Autodesk Inventor part; units mm, degrees
ref_plane "YZ Plane" through (0, 0, 0) normal (1, 0, 0) x (0, 1, 0)
ref_plane "XZ Plane" through (0, 0, 0) normal (0, 1, 0) x (-1, 0, 0)
ref_plane "XY Plane" through (0, 0, 0) normal (0, 0, 1) x (1, 0, 0)
sketch "Sketch1" plane through (0, 0, 0) normal (0, 0, 1) x (1, 0, 0)
  line L0 (-18.671, 23.6638) -> (26.829, 23.6638)
  line L1 (26.829, 23.6638) -> (26.829, -28.3362)
  line L2 (26.829, -28.3362) -> (-18.671, -28.3362)
  line L3 (-18.671, -28.3362) -> (-18.671, 23.6638)
  point P0 (0, 0)
  dimension "d0" = 52
  dimension "d1" = 45.5
extrude "Extrusion1" add sketch "Sketch1" along normal blind 2
sketch "Sketch2" plane through (0, 0, 2) normal (0, 0, 1) x (1, 0, 0)
  line L0 (-18.671, -28.3362) -> (26.829, -28.3362)
  line L1 (26.829, -28.3362) -> (26.829, 23.6638)
  line L2 (26.829, 23.6638) -> (-18.671, 23.6638)
  point P0 (0, 0)
  point P1 (-13.171, 20.6638)
  point P2 (21.829, 20.6638)
  point P3 (21.829, -25.3362)
  point P4 (-13.171, -25.3362)
  point P5 (23.829, -28.3362)
  point P6 (26.829, -25.3362)
  point P7 (26.829, 20.6638)
  point P8 (23.829, 23.6638)
  dimension "d5" = 35
  dimension "d6" = 35
  dimension "d7" = 46
  dimension "d8" = 3
  dimension "d9" = 3
  dimension "d10" = 5
  dimension "d11" = 5
  dimension "d12" = 3
hole "Hole1" at (-13.171, 20.6638, 2) at (21.829, 20.6638, 2) at (21.829, -25.3362, 2) at (-13.171, -25.3362, 2) direction (0, 0, -1) diameter 3.2 depth 10 tip angle 118
sketch "Sketch3" plane through (0, 0, 2) normal (0, 0, 1) x (1, 0, 0)
  line L0 (-18.671, 23.6638) -> (-18.671, -28.3362)
  line L1 (-18.671, 15.6638) -> (20.829, 15.6638)
  line L2 (20.829, 15.6638) -> (20.829, -20.3362)
  line L3 (20.829, -20.3362) -> (-18.671, -20.3362)
  line L4 (-18.671, -20.3362) -> (-18.671, 15.6638)
  circle A0 centre (-13.171, 20.6638) radius 1.6
  line L5 (26.829, -28.3362) -> (26.829, 23.6638)
  circle A1 centre (-13.171, -25.3362) radius 1.6
  point P0 (0, 0)
  point P1 (26.829, -25.3362)
  point P2 (26.829, 20.6638)
  dimension "d20" = 5
  dimension "d21" = 6
  dimension "d22" = 5
extrude "Extrusion2" cut sketch "Sketch3" against normal blind 2 contours L1 L2 L3 L0
sketch "Sketch4" plane through (0, 0, 2) normal (0, 0, 1) x (1, 0, 0)
  line L0 (-18.671, 15.6638) -> (20.829, 15.6638)
  line L1 (-18.671, 15.6638) -> (-13.671, 15.6638)
  line L2 (-13.671, 15.6638) -> (-13.671, 7.6638)
  line L3 (-13.671, 7.6638) -> (-18.671, 7.6638)
  line L4 (-18.671, 7.6638) -> (-18.671, 15.6638)
  line L5 (-18.671, -20.3362) -> (-18.671, -28.3362)
  line L6 (-18.671, -20.3362) -> (-13.671, -20.3362)
  line L7 (-13.671, -20.3362) -> (-13.671, -12.3362)
  line L8 (-13.671, -12.3362) -> (-18.671, -12.3362)
  line L9 (-18.671, -12.3362) -> (-18.671, -20.3362)
  point P0 (0, 0)
  point P1 (17.829, 15.6638)
  point P2 (-18.671, -25.3362)
  dimension "d27" = 8
  dimension "d28" = 8
  dimension "d29" = 5
extrude "Extrusion3" add sketch "Sketch4" against normal blind 2
fillet "Fillet5" radius 2 4 edges at (-13.671, 7.6638, 1) (-18.671, 7.6638, 1) (-18.671, -12.3362, 1) (-13.671, -12.3362, 1)
sketch "Sketch5" plane through (0, 0, 2) normal (0, 0, 1) x (1, 0, 0)
  line L0 (26.829, 23.6638) -> (-18.671, 23.6638)
  line L1 (-18.671, 23.6638) -> (26.829, 23.6638)
  line L2 (26.829, 23.6638) -> (26.829, 24.1638)
  line L3 (26.829, 24.1638) -> (-18.671, 24.1638)
  line L4 (-18.671, 24.1638) -> (-18.671, 23.6638)
  line L5 (-18.671, -28.3362) -> (26.829, -28.3362)
  line L6 (-18.671, -28.3362) -> (26.829, -28.3362)
  line L7 (26.829, -28.3362) -> (26.829, -28.8362)
  line L8 (26.829, -28.8362) -> (-18.671, -28.8362)
  line L9 (-18.671, -28.8362) -> (-18.671, -28.3362)
  line L10 (26.829, -28.3362) -> (26.829, 23.6638)
  point P0 (0, 0)
  dimension "d37" = 0.5
  dimension "d38" = 0.5
extrude "Extrusion4" add sketch "Sketch5" against normal blind 2
fillet "Fillet6" radius 3 4 edges at (-18.671, 24.1638, 1) (26.829, 24.1638, 1) (26.829, -28.8362, 1) (-18.671, -28.8362, 1)
chamfer "Chamfer2" distance 3 angle 45 4 edges at (-13.671, 15.6638, 1) (20.829, 15.6638, 1) (-13.671, -20.3362, 1) (20.829, -20.3362, 1)
sketch "Sketch6" plane through (0, 0, 2) normal (0, 0, 1) x (1, 0, 0)
  circle A0 centre (-13.171, -25.3362) radius 1.6
  circle A1 centre (-13.171, 20.6638) radius 1.6
  circle A2 centre (21.829, 20.6638) radius 1.6
  line L0 (23.829, 24.1638) -> (-15.671, 24.1638)
  line L1 (-15.671, -28.8362) -> (23.829, -28.8362)
  circle A3 centre (21.829, -25.3362) radius 1.6
  point P0 (0, 0)
  dimension "d46" = 46
  dimension "d47" = 35
  dimension "d48" = 3.5
  dimension "d49" = 3.5
  dimension "d50" = 3.5
  dimension "d51" = 3.5
properties part number "wood_supp"
Can you work these out from the model? Positions are in its coordinate system, mm. A direction names the side the tool comes from. Round coordinates to 2 decimals unless told otherwise and drop trailing zeros. Order: outer loops, then holes, each group sorted by start corner. A loop starts at its lowest first (then second) coordinate and runs counter-clockwise, first axis right, second up. Notation, with made-up numbers: (86.25, 60) -> (98.25, 60) arc R23 ccw to (98.25, 72) -> close; hole circle Ø1 at (-27.5, -20.75). An arc over 180 degrees is marked (long way). Return JSON: item names as keys, results as strings. Group by question number.
1. We'd pull the mould along X, two halves only. Please class faces 1 (the face through (22.803, 21.934, 0.986)), 2 (the face through (26.829, -2, 1)), 3 (the face through (4, 24.164, 1)): released by +X, released by -X, zero draft, split by the parting line, or undercut.
2. I need wall thicknesses on line 1 (Y direction, x = 8, z = 0.3); line 2 (Y direction, x = -15.5, z = 0.15); line 3 (X direction, y = 12, z = 0.85). Which ranges of each line are inside material? Lowest first, please. Write a range as [from, to].
3. If we section it at D-D, the plane y = 2: Write out the boundary of the cut face in (x, z), then the cut area to 3 significant figures.
4. If we section it at C-C, the plane z = 0.4: Write out the boundary of the cut face in (x, y), then the cut area to 3 significant figures.
5. Which directions (+Z, -Z, +X, -X, +Y, -Y) give clear straight access to the entire face, cutting with the end or side of a thin tool? Please do faces 4 (the face through (4, -20.336, 1)), 5 (the face through (4, 16, 2)).
6. If we section it at A-A, the plane x = 7: Write out the boundary of the cut face in (y, z).
7. If we section it at B-B, the plane y = 20: Write out the boundary of the cut face in (x, z).
8. Will these pins go through, and if not, where does the flat tip stop? pin 1 (1 mm diameter, centred on y = -2.5, z = 0.5, fed in from -X); pin 2 (1.9 mm diameter, centred on x = -13.17, y = 20.66, fed in from +Z).
Output values:
{
 "1": {"face 1": "undercut", "face 2": "released by +X", "face 3": "zero draft"},
 "2": {"line 1": "[-28.84, -20.34], [15.66, 24.16]", "line 2": "[-28.84, -12.34], [7.67, 24.16]", "line 3": "[-18.67, -13.67], [20.83, 26.83]"},
 "3": {"outline": "(20.83, 0) -> (26.83, 0) -> (26.83, 2) -> (20.83, 2) -> close", "area": "12.0 mm²"},
 "4": {"outline": "(-18.67, -25.84) arc R3 ccw to (-15.67, -28.84) -> (23.83, -28.84) arc R3 ccw to (26.83, -25.84) -> (26.83, 21.16) arc R3 ccw to (23.83, 24.16) -> (-15.67, 24.16) arc R3 ccw to (-18.67, 21.16) -> (-18.67, 9.66) arc R2 ccw to (-16.67, 7.66) -> (-15.67, 7.66) arc R2 ccw to (-13.67, 9.66) -> (-13.67, 12.66) -> (-10.67, 15.66) -> (17.83, 15.66) -> (20.83, 12.66) -> (20.83, -17.34) -> (17.83, -20.34) -> (-10.67, -20.34) -> (-13.67, -17.34) -> (-13.67, -14.34) arc R2 ccw to (-15.67, -12.34) -> (-16.67, -12.34) arc R2 ccw to (-18.67, -14.34) -> close; hole circle Ø3.2 at (-13.17, -25.34); hole circle Ø3.2 at (-13.17, 20.66); hole circle Ø3.2 at (21.83, -25.34); hole circle Ø3.2 at (21.83, 20.66)", "area": "1,040 mm²"},
 "5": {"face 4": "+Z, -Z", "face 5": "+Z, +X, -X, +Y, -Y"},
 "6": {"outline": "(-28.84, 0) -> (-20.34, 0) -> (-20.34, 2) -> (-28.84, 2) -> close; (15.66, 0) -> (24.16, 0) -> (24.16, 2) -> (15.66, 2) -> close"},
 "7": {"outline": "(-18.67, 0) -> (-14.63, 0) -> (-14.63, 2) -> (-18.67, 2) -> close; (-11.72, 0) -> (20.37, 0) -> (20.37, 2) -> (-11.72, 2) -> close; (23.28, 0) -> (26.83, 0) -> (26.83, 2) -> (23.28, 2) -> close"},
 "8": {"pin 1": "x = 20.83", "pin 2": "through"}
}
